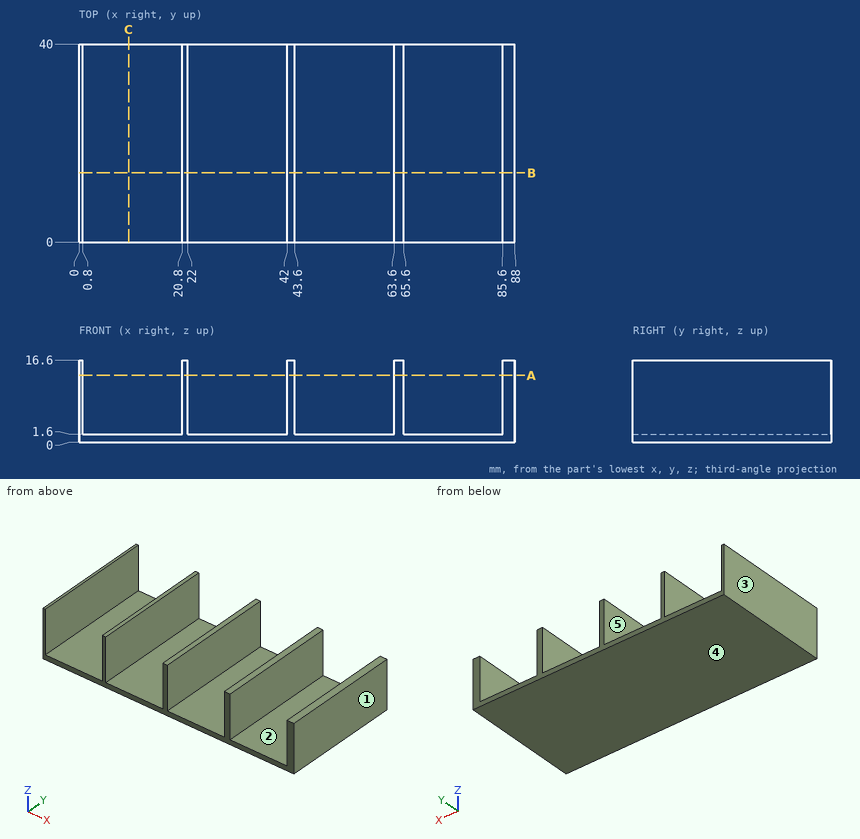
Part print with two shaded views. Sizes in mm from the minimum x, y, z corner. A direction names the side the tool comes from. Coordinates: 2 decimals unless noted, no trailing zeros. Write each loop counter-clockwise with the first axis right and the second up, starting at its lowest first coordinate (ties: lowest second). Pieces come first, ordered by that corner, then holes.
1. Band-saw the part on A-A, the plane z = 13.5. Give the cut face in (x, y).
Answer block:
outline: (0, 0) - (0.8, 0) - (0.8, 40) - (0, 40) - close; (20.8, 0) - (22, 0) - (22, 40) - (20.8, 40) - close; (42, 0) - (43.6, 0) - (43.6, 40) - (42, 40) - close; (63.6, 0) - (65.6, 0) - (65.6, 40) - (63.6, 40) - close; (85.6, 0) - (88, 0) - (88, 40) - (85.6, 40) - close
2. Pull direction X, two halves, no side cores. Call the marked faces 3, 4 and 5: released by +X, released by -X, zero draft, split by the parting line, or undercut.
Answer block:
face 3: released by -X
face 4: zero draft
face 5: undercut
3. 3-axis set-ups, long thin cutter, end or side, ignore diameter. For the marked faces 1 and 2: which of +Z, -Z, +X, -X, +Y, -Y reach the whole face in a straight line?
Answer block:
face 1: +Z, -Z, +X, +Y, -Y
face 2: +Z, +Y, -Y
4. Band-saw the part on C-C, the plane x = 10. Give the cut face in (y, z), and give its area (3 significant figures).
Answer block:
outline: (0, 0) - (40, 0) - (40, 1.6) - (0, 1.6) - close
area: 64.0 mm2
5. Drop flat-ended pins along their axis: pin 1 (6 mm diameter, centred on x = 38.5, y = 24.5, fed in from +Z); pin 2 (3 mm diameter, centred on y = 6.5, z = 9, fed in from -X). Give the stop position or say it passes through.
Answer block:
pin 1: stops at z = 1.6
pin 2: stops at x = 0
6. Drill centre lines: probe 1 along X at (y, z) = (7, 12); probe 2 along Z at (x, y) = (48, 12). Where is each one in solid material? Low to high.
Answer block:
probe 1: x = 0 to 0.8, 20.8 to 22, 42 to 43.6, 63.6 to 65.6, 85.6 to 88
probe 2: z = 0 to 1.6
7. Band-saw the part on B-B, the plane y = 14. Give the cut face in (x, z), and give its area (3 significant figures).
Answer block:
outline: (0, 0) - (88, 0) - (88, 16.6) - (85.6, 16.6) - (85.6, 1.6) - (65.6, 1.6) - (65.6, 16.6) - (63.6, 16.6) - (63.6, 1.6) - (43.6, 1.6) - (43.6, 16.6) - (42, 16.6) - (42, 1.6) - (22, 1.6) - (22, 16.6) - (20.8, 16.6) - (20.8, 1.6) - (0.8, 1.6) - (0.8, 16.6) - (0, 16.6) - close
area: 261 mm2
